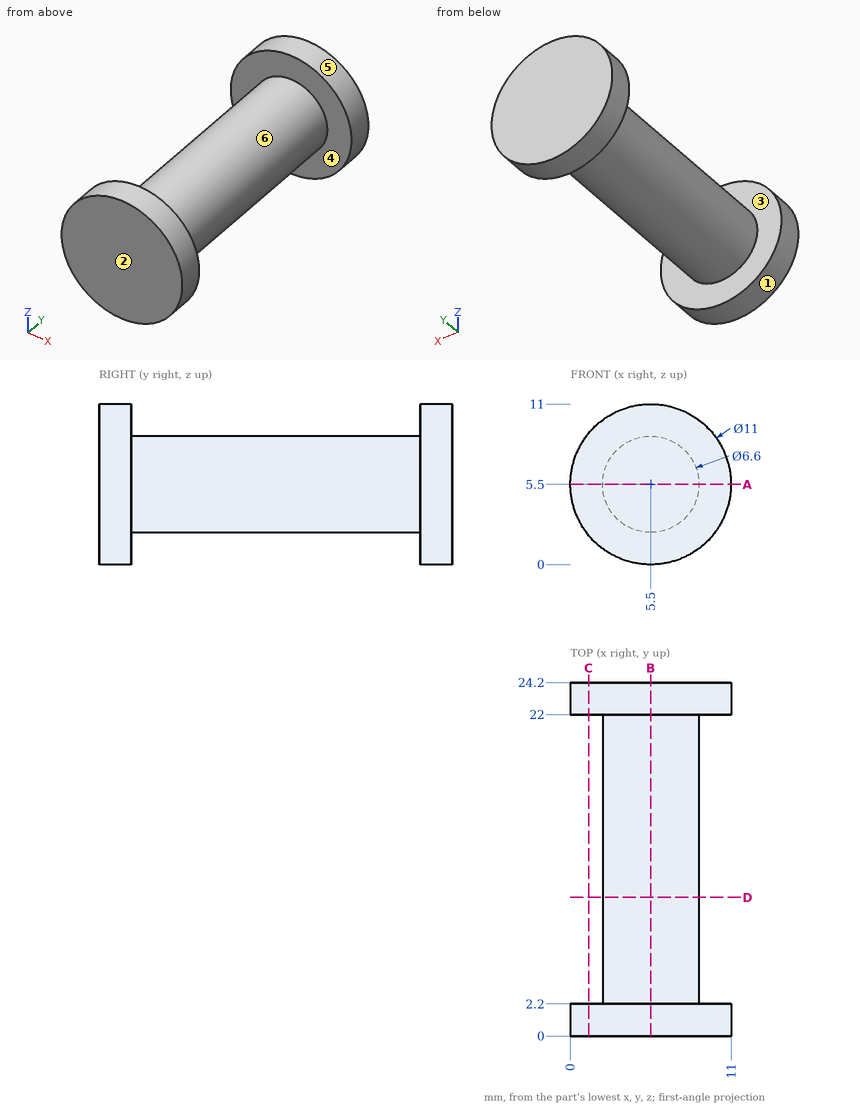
The figure shows three views and two pictorial views of one solid part (mm, origin at its lowest corner). Answer the questions. A direction names the side the tool comes from. Coordinates: 2 decimals unless noted, no trailing zeros. Write each loop counter-clockwise with the first axis right and the second up, starting at its lowest first coordinate (ties: lowest second). Pieces come first, ordered by that corner, then holes. Notation, with made-up numbers: (60, -34.5) -> (66, -34.5) arc R12 cw to (66, -13.5) -> close; hole circle Ø6 at (24, 44). An arc over 180 degrees is marked (long way). Answer as a JSON object with one key per item and string values.
Q1. The part is cut by section B-B on x = 5.5. Give the vertices of the cut face in (y, z).
The answers:
{"outline": "(0, 0) -> (2.2, 0) -> (2.2, 2.2) -> (22, 2.2) -> (22, 0) -> (24.2, 0) -> (24.2, 11) -> (22, 11) -> (22, 8.8) -> (2.2, 8.8) -> (2.2, 11) -> (0, 11) -> close"}
Q2. Consider line 1 (Y direction, x = 1, z = 7.25); line 2 (X direction, y = 9.5, z = 5.5); line 3 (Z direction, x = 3.5, y = 2). Determine where each line is inside the solid, lowest interval first. Write a range as [from, to].
The answers:
{"line 1": "y = [0, 2.2], [22, 24.2]", "line 2": "x = [2.2, 8.8]", "line 3": "z = [0.38, 10.62]"}
Q3. The part is cut by section C-C on x = 1.25. Give the vertices of the cut face in (y, z), then the cut area to 3 significant figures.
The answers:
{"outline": "(0, 2.01) -> (2.2, 2.01) -> (2.2, 8.99) -> (0, 8.99) -> close; (22, 2.01) -> (24.2, 2.01) -> (24.2, 8.99) -> (22, 8.99) -> close", "area": "30.7 mm2"}
Q4. The part is cut by section D-D on y = 9.5. Give the vertices of the cut face in (x, z), then the cut area to 3 significant figures.
The answers:
{"outline": "circle Ø6.6 at (5.5, 5.5)", "area": "34.2 mm2"}
Q5. A tool of negligible diameter and unlimited length cuts with its end or side. For the marked faces 5 and 6, from which of +Z, -Z, +X, -X, +Y, -Y can it reach the whole face along a straight path? Write none if from no direction.
The answers:
{"face 5": "+Y, -Y", "face 6": "none"}
Q6. Determine the mould class of the marked faces 1, 2, 3 and 4 for opening direction Y: pulls with the +Y half, pulls with the -Y half, needs draft (parallel to the pull), parting line crosses it, or undercut.
The answers:
{"face 1": "needs draft", "face 2": "pulls with the -Y half", "face 3": "undercut", "face 4": "undercut"}
Q7. The part is cut by section A-A on z = 5.5. Give the vertices of the cut face in (x, y), then the cut area to 3 significant figures.
The answers:
{"outline": "(0, 0) -> (11, 0) -> (11, 2.2) -> (8.8, 2.2) -> (8.8, 22) -> (11, 22) -> (11, 24.2) -> (0, 24.2) -> (0, 22) -> (2.2, 22) -> (2.2, 2.2) -> (0, 2.2) -> close", "area": "179 mm2"}
Q8. Flat-ended cylindrical pins translate along their axes: pin 1 Ø3 at (x, y) = (2, 9) entering from -Z; pin 2 Ø4 at (y, z) = (5, 8.5) entering from -X; pin 3 Ø6 at (y, z) = (6, 2.5) entering from +X. Find the tip coordinate at first contact, or state that the pin passes through.
The answers:
{"pin 1": "stops at z = 2.88", "pin 2": "stops at x = 2.36", "pin 3": "stops at x = 8.8"}
